CAD build for the part. Positions are in the model's coordinates, mm. Round coordinates to 2 decimals unless told otherwise and drop trailing zeros. Order: outer loops, then holes, each group sorted by start corner. A loop starts at its lowest first (then second) coordinate and runs counter-clockwise, first axis right, second up.
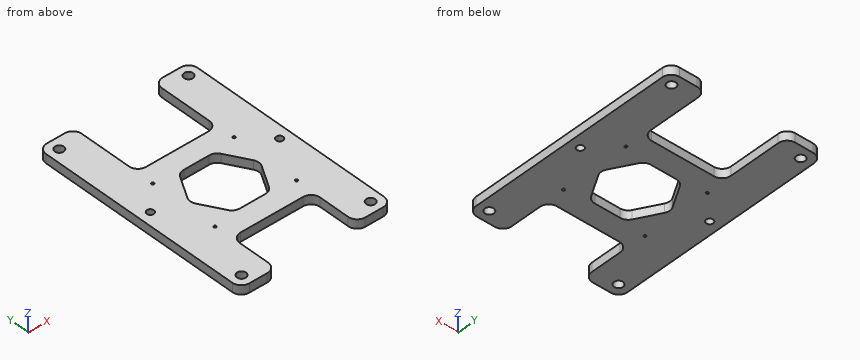
```python
from build123d import *

# Parameters (mm, degrees)
SKETCH1_R           = 0.889
SKETCH1_R_2         = 3.175
SKETCH1_R_3         = 2.45745
BOSS_EXTRUDE1_DEPTH = 6.35
FILLET3_R           = 6.35


with BuildPart() as part:
    # Sketch1 → Boss-Extrude1 (new body)
    with BuildSketch(Plane.XY):
        Polygon((-53.975, -79.509375), (-53.975, 79.509375), (-28.575, 79.509375), (-28.575, 29.7), (28.575, 29.7), (28.575, 79.509375), (53.975, 79.509375), (53.975, -79.509375), (28.575, -79.509375), (28.575, -44.7), (-28.575, -44.7), (-28.575, -79.509375), align=None)
        with Locations((29, 17)):
            Circle(SKETCH1_R, mode=Mode.SUBTRACT)
        with Locations((29, -32)):
            Circle(SKETCH1_R, mode=Mode.SUBTRACT)
        with Locations((-29, -32)):
            Circle(SKETCH1_R, mode=Mode.SUBTRACT)
        with Locations((-29, 17)):
            Circle(SKETCH1_R, mode=Mode.SUBTRACT)
        with Locations((-46.0375, 71.571875)):
            Circle(SKETCH1_R_2, mode=Mode.SUBTRACT)
        with Locations(Location((46.0375, 71.571875, 0), (0, 0, 180))):
            Circle(SKETCH1_R_2, mode=Mode.SUBTRACT)
        with Locations(Location((-46.0375, -71.571875, 0), (0, 0, 180))):
            Circle(SKETCH1_R_2, mode=Mode.SUBTRACT)
        with Locations((46.0375, -71.571875)):
            Circle(SKETCH1_R_2, mode=Mode.SUBTRACT)
        with Locations((-46.0375, 0)):
            Circle(SKETCH1_R_3, mode=Mode.SUBTRACT)
        with Locations((46.0375, 0)):
            Circle(SKETCH1_R_3, mode=Mode.SUBTRACT)
        Polygon((-12.7, -29.497045256), (12.7, -29.497045256), (25.4, -7.5), (12.7, 14.497045256), (-12.7, 14.497045256), (-25.4, -7.5), align=None, mode=Mode.SUBTRACT)
    extrude(amount=BOSS_EXTRUDE1_DEPTH)

    # Fillet3
    fillet3_edges = [part.edges().sort_by_distance(p)[0] for p in [
        (-53.975, -79.509375, 3.175),
        (-53.975, 79.509375, 3.175),
        (-28.575, 79.509375, 3.175),
        (-28.575, 29.7, 3.175),
        (28.575, 29.7, 3.175),
        (28.575, 79.509375, 3.175),
        (53.975, 79.509375, 3.175),
        (53.975, -79.509375, 3.175),
        (28.575, -79.509375, 3.175),
        (28.575, -44.7, 3.175),
        (-28.575, -44.7, 3.175),
        (-28.575, -79.509375, 3.175),
        (-25.4, -7.5, 3.175),
        (-12.7, -29.497045256, 3.175),
        (12.7, -29.497045256, 3.175),
        (25.4, -7.5, 3.175),
        (12.7, 14.497045256, 3.175),
        (-12.7, 14.497045256, 3.175),
    ]]
    fillet(fillet3_edges, radius=FILLET3_R)


solid = part.part
```
1. Cut at B-B, the plane y = 51.5. Write the cut outline in (x, z) (3 decimals).
2. Drill centre lines: line 1 (X direction, y = 40, z = 5) (3 decimals); line 2 (Y direction, x = -9.5, z = 1.5); line 3 (X direction, y = -6, z = 4.5) (3 decimals). Where is each one in solid material? Low to high.
3. Cut at A-A, the plane x = 0.5. Write the cut outline in (y, z).
4. Pin check, flat tips, straight feed: P1, Ø6.5, axis at x = -46.04, y = 0, coming from the +Z side; P2, Ø3, axis at x = -1.5, z = 4, coming from the +Y side; P3, Ø1.1, axis at x = 29, y = 17, coming from the +Z side; P4, Ø3, axis at x = 2.5, z = 3.5, coming from the -Y side. Stop position of each tip, or through.
5. Cut at D-D, the plane z = 3.5. Give the number of separate pieces and of enclosed holes in the cut face, and give its area (3 significant figures).
6. Cut at C-C, the plane y = 0. Write the cut outline in (x, z) (3 decimals).
Outcome:
1. outline: (-53.975, 0) - (-28.575, 0) - (-28.575, 6.35) - (-53.975, 6.35) - close; (28.575, 0) - (53.975, 0) - (53.975, 6.35) - (28.575, 6.35) - close
2. line 1: x = -53.975 to -28.575, 28.575 to 53.975
2. line 2: y = -44.7 to -29.48, 14.48 to 29.7
2. line 3: x = -53.975 to -24.238, 24.238 to 53.975
3. outline: (-44.7, 0) - (-29.5, 0) - (-29.5, 6.35) - (-44.7, 6.35) - close; (14.5, 0) - (29.7, 0) - (29.7, 6.35) - (14.5, 6.35) - close
4. P1: stops at z = 6.35
4. P2: stops at y = 29.7
4. P3: passes through
4. P4: stops at y = -44.7
5. separate pieces: 1
5. enclosed holes: 11
5. area: 10,500 mm2
6. outline: (-53.975, 0) - (-48.495, 0) - (-48.495, 6.35) - (-53.975, 6.35) - close; (-43.58, 0) - (-21.07, 0) - (-21.07, 6.35) - (-43.58, 6.35) - close; (21.07, 0) - (43.58, 0) - (43.58, 6.35) - (21.07, 6.35) - close; (48.495, 0) - (53.975, 0) - (53.975, 6.35) - (48.495, 6.35) - close
